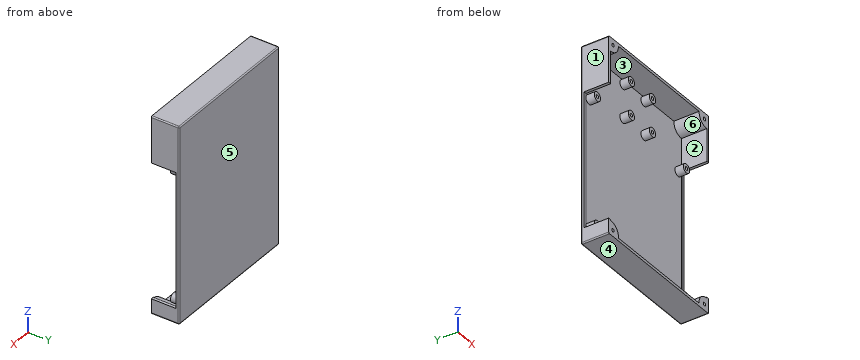
from build123d import *

# Parameters (mm, degrees)
F1_W      = 128
F1_H      = 175
F2_DEPTH  = 25
F3_T      = -2.5
F4_R      = 4
F4_R_2    = 1.5
F5_DEPTH  = 10
F7_W      = 6.963276
F7_H      = 120.338105
F8_DEPTH  = 35
F9_R      = 1.5
F10_DEPTH = 25
F11_R     = 1


with BuildPart() as f2:
    # F1 (on Front) → F2 (new body)
    with BuildSketch(Plane.XZ):
        with Locations((0, 36.5)):
            Rectangle(F1_W, F1_H)
    extrude(amount=F2_DEPTH)

    # F3
    f3_openings = [f2.faces().sort_by_distance(p)[0] for p in [
        (0, -25, 36.5),
    ]]
    offset(amount=F3_T, openings=f3_openings)

    # F4 (on Front) → F5 (join)
    with BuildSketch(Plane.XZ):
        with Locations((-57, 79.671152)):
            Circle(F4_R)
        with Locations((-57, 79.671152)):
            Circle(F4_R_2, mode=Mode.SUBTRACT)
        with Locations((57, 79.671152)):
            Circle(F4_R)
        with Locations((57, 79.671152)):
            Circle(F4_R_2, mode=Mode.SUBTRACT)
        with Locations((57, -34.24717)):
            Circle(F4_R)
        with Locations((57, -34.24717)):
            Circle(F4_R_2, mode=Mode.SUBTRACT)
        with Locations((-57, -34.328848)):
            Circle(F4_R)
        with Locations((-57, -34.328848)):
            Circle(F4_R_2, mode=Mode.SUBTRACT)
        with Locations((-13.5, 117.413834)):
            Circle(F4_R)
        with Locations((-13.5, 117.413834)):
            Circle(F4_R_2, mode=Mode.SUBTRACT)
        with Locations((13.5, 117.413834)):
            Circle(F4_R)
        with Locations((13.5, 117.413834)):
            Circle(F4_R_2, mode=Mode.SUBTRACT)
        with Locations((-13.5, 87.413834)):
            Circle(F4_R)
        with Locations((-13.5, 87.413834)):
            Circle(F4_R_2, mode=Mode.SUBTRACT)
        with Locations((13.5, 87.413834)):
            Circle(F4_R)
        with Locations((13.5, 87.413834)):
            Circle(F4_R_2, mode=Mode.SUBTRACT)
    extrude(amount=F5_DEPTH)

    # F7 (on offset) → F8 (cut)
    with BuildSketch(Plane.XZ.offset(3)):
        with Locations((-64.73311, 22.50288)):
            Rectangle(F7_W, F7_H)
        with Locations((64.73311, 22.50288)):
            Rectangle(F7_W, F7_H)
    extrude(amount=F8_DEPTH, mode=Mode.SUBTRACT)

    # F9 (on Front) → F10 (join)
    with BuildSketch(Plane.XZ):
        with BuildLine():
            Line((-61.5, -38.5), (-61.5, -48.5))
            Line((-61.5, -48.5), (-51.5, -48.5))
            ThreePointArc((-51.5, -48.5), (-54.260082, -41.260082), (-61.5, -38.5))
        make_face()
        with Locations((-58.5, -45.5)):
            Circle(F9_R, mode=Mode.SUBTRACT)
        with BuildLine():
            ThreePointArc((61.5, -38.5), (54.260082, -41.260082), (51.5, -48.5))
            Line((51.5, -48.5), (61.5, -48.5))
            Line((61.5, -48.5), (61.5, -38.5))
        make_face()
        with Locations((58.5, -45.5)):
            Circle(F9_R, mode=Mode.SUBTRACT)
        with BuildLine():
            ThreePointArc((-61.645352, 111.683935), (-54.405433, 114.444017), (-51.645352, 121.683935))
            Line((-51.645352, 121.683935), (-61.645352, 121.683935))
            Line((-61.645352, 121.683935), (-61.645352, 111.683935))
        make_face()
        with Locations((-58.5, 118.5)):
            Circle(F9_R, mode=Mode.SUBTRACT)
        with BuildLine():
            Line((61.645352, 111.683935), (61.645352, 121.683935))
            Line((61.645352, 121.683935), (51.645352, 121.683935))
            ThreePointArc((51.645352, 121.683935), (54.405433, 114.444017), (61.645352, 111.683935))
        make_face()
        with Locations((58.5, 118.5)):
            Circle(F9_R, mode=Mode.SUBTRACT)
    extrude(amount=F10_DEPTH)

    # F11
    f11_edges = [f2.edges().sort_by_distance(p)[0] for p in [
        (-64, -12.5, 124),
        (64, -12.5, 124),
        (0, 0, 124),
        (64, 0, 36.5),
        (0, 0, -51),
        (64, -12.5, -51),
        (-64, -12.5, -51),
        (-64, 0, 36.5),
    ]]
    fillet(f11_edges, radius=F11_R)


solid = f2.part
Read the model definition and answer for the solid it produces. Units are mm, in the model's axes. Face numbers are marked on the shaded views. A direction names the side the tool comes from. Round coordinates to 2 decimals unless told otherwise and drop trailing zeros. Write each loop counter-clockwise with the first axis right and the second up, starting at its lowest first coordinate (ties: lowest second). Pieces come first, ordered by that corner, then holes. Notation, with made-up numbers: (-9, 55.5) - (37, 55.5) arc R29 cw to (37, 80.5) - close; hole circle Ø2 at (-21.5, -22.5). An arc over 180 degrees is marked (long way). Use a Markdown table: item, result.
(1) The part is cut by section A-A (y = -19.75). Write down the section's boundary in (x, z), then the cut area to 3 significant figures.
Reported:
| item | result |
|---|---|
| outline | (-64, -50) arc R1 ccw to (-63, -51) - (63, -51) arc R1 ccw to (64, -50) - (64, -37.67) - (61.5, -37.67) - (61.5, -38.5) arc R9.48 ccw to (51.5, -48.5) - (-51.5, -48.5) arc R9.48 ccw to (-61.5, -38.5) - (-61.5, -37.67) - (-64, -37.67) - close; (-64, 82.67) - (-61.5, 82.67) - (-61.5, 111.68) arc R9.48 ccw to (-51.64, 121.5) - (51.64, 121.5) arc R9.48 ccw to (61.5, 111.68) - (61.5, 82.67) - (64, 82.67) - (64, 123) arc R1 ccw to (63, 124) - (-63, 124) arc R1 ccw to (-64, 123) - close; hole circle Ø3 at (-58.5, -45.5); hole circle Ø3 at (-58.5, 118.5); hole circle Ø3 at (58.5, -45.5); hole circle Ø3 at (58.5, 118.5) |
| area | 1,180 mm2 |
(2) Which of the six approach directions +Z, -Z, +X, -X, +Y, -Y give full straight-line access (tool end or side, diameter ignored) to the marked faces 1 and 2?
Reported:
| item | result |
|---|---|
| face 1 | +Z, -Z, -X, +Y, -Y |
| face 2 | -Y |
(3) The mould has two halves that part along Z. Classify the marked faces 3, 4, 5 and 6: released by +Z, released by -Z, zero draft, split by the parting line, or undercut.
Reported:
| item | result |
|---|---|
| face 3 | undercut |
| face 4 | released by -Z |
| face 5 | zero draft |
| face 6 | undercut |
(4) The part is cut by section C-C (x = -48). Write down the section's boundary in (y, z), then the cut area to 3 significant figures.
Reported:
| item | result |
|---|---|
| outline | (-25, -51) - (-1, -51) arc R1 ccw to (0, -50) - (0, 123) arc R1 ccw to (-1, 124) - (-25, 124) - (-25, 121.5) - (-2.5, 121.5) - (-2.5, -48.5) - (-25, -48.5) - close |
| area | 550 mm2 |
(5) The part is cut by section D-D (y = -4.75). State how many separate pieces and enclosed holes the cut face has, then the cut area to 3 significant figures.
Reported:
| item | result |
|---|---|
| separate pieces | 10 |
| enclosed holes | 12 |
| area | 1,520 mm2 |
(6) Straight lines are drawn through the part: line 1 along Z through (x, y) = (-32, -23); line 2 along X through (y, z) = (-12.25, 118.5); line 3 along X through (y, z) = (-20.5, 93). For each, find the intervals that lie inside material, in ascending order. Write a range as [from, to].
Reported:
| item | result |
|---|---|
| line 1 | [-51, -48.5], [121.5, 124] |
| line 2 | [-64, -60], [-57, -52.01], [52.01, 57], [60, 64] |
| line 3 | [-64, -61.5], [61.5, 64] |
(7) Each of these flat-tipped pins is pushed along its axis until it touches: pin 1 Ø4 at (x, z) = (55.5, -33) entering from -Y; pin 2 Ø2.5 at (x, z) = (-13.5, 87.41) entering from -Y; pin 3 Ø3 at (x, z) = (-63, 0.5) entering from -Y. Where does it stop, or does it pass through?
Reported:
| item | result |
|---|---|
| pin 1 | y = -10 |
| pin 2 | y = -2.5 |
| pin 3 | y = -3 |
(8) The part is cut by section B-B (z = -5). Write down the section's boundary in (x, y).
Reported:
| item | result |
|---|---|
| outline | (-64, -3) - (-61.5, -3) - (-61.5, -2.5) - (61.5, -2.5) - (61.5, -3) - (64, -3) - (64, -1) arc R1 ccw to (63, 0) - (-63, 0) arc R1 ccw to (-64, -1) - close |
